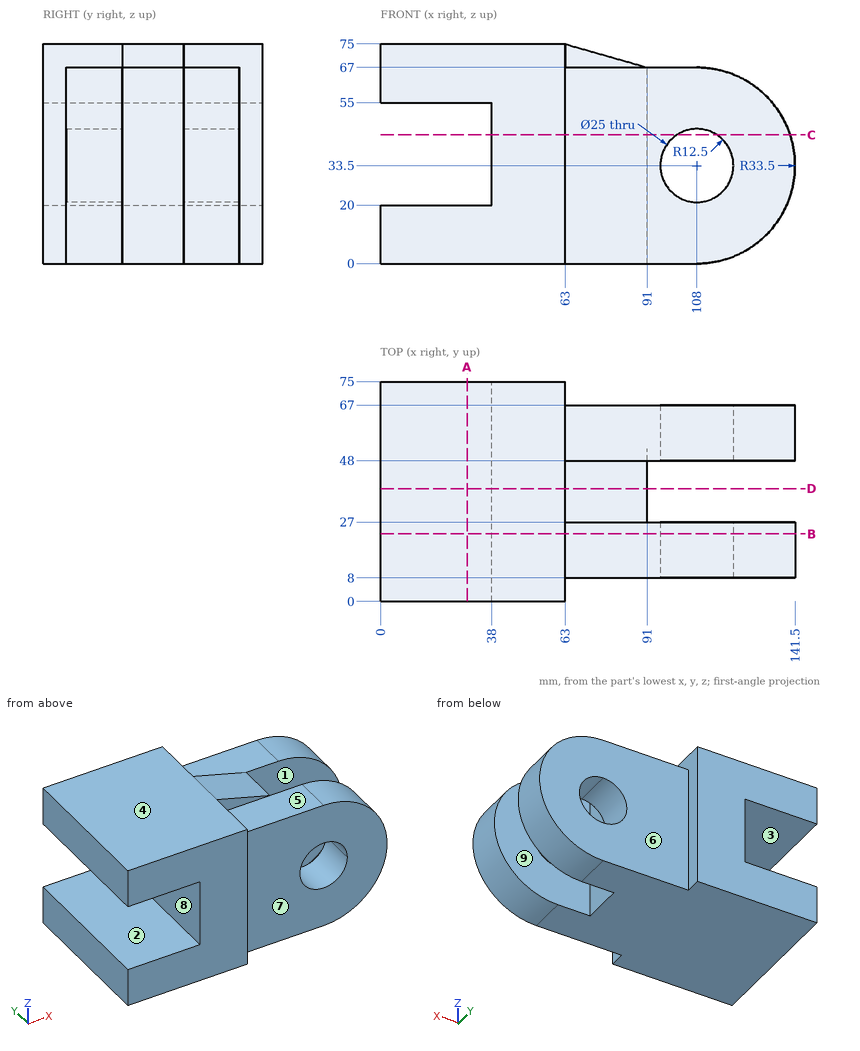
Job drawing, mm, ordinate dimensions from the low corner. One solid piece. A direction names the side the tool comes from. Round coordinates to 2 decimals unless told otherwise and drop trailing zeros. Loops run counter-clockwise (first coordinate to the right, second up) from the corner with the lowest first, then second, coordinate; pieces in that order, holes last.
Item 1: Cut at A-A, the plane x = 29.5. Give the cut face in (y, z), then the cut area to 3 significant figures.
Item 2: Cut at D-D, the plane y = 38.5. Give the cut face in (x, z), then the cut area to 3 significant figures.
Item 3: Mould opens along Z. For the marked faces 1, 2, 3 and 4 say: +Z half, -Z half, draft (parallel to the pull), parting line (faces both ways), or undercut.
Item 4: Drill centre lines: line 1 (Z direction, x = 8, y = 41.5); line 2 (Z direction, x = 108, y = 62); line 3 (Y direction, x = 97, z = 64). Where is each one in solid material? Low to high.
Item 5: Cut at C-C, the plane z = 44. Give the cut face in (x, y), then the cut area to 3 significant figures.
Item 6: Drop flat-ended pins along their axis: P1, Ø6, axis at y = 12, z = 33, coming from the -X side; P2, Ø21.5, axis at y = 65.5, z = 44.5, coming from the +X side; P3, Ø21, axis at x = 88, y = 17, coming from the +Z side; P4, Ø15, axis at x = 108, z = 33.5, coming from the +Y side. Give the stop position or say it passes through.
Item 7: 3-axis set-ups, long thin cutter, end or side, ignore diameter. For the marked faces 5, 6, 7, 8 and 9: which of +Z, -Z, +X, -X, +Y, -Y reach the whole face in a straight line?
Item 8: Cut at B-B, the plane y = 23. Give the cut face in (x, z), then the cut area to 3 significant figures.
A:
1. outline: (0, 0) - (75, 0) - (75, 20) - (0, 20) - close; (0, 55) - (75, 55) - (75, 75) - (0, 75) - close
1. area: 3,000 mm2
2. outline: (0, 0) - (91, 0) - (91, 67) - (63, 75) - (0, 75) - (0, 55) - (38, 55) - (38, 20) - (0, 20) - close
2. area: 5,380 mm2
3. face 1: draft
3. face 2: undercut
3. face 3: undercut
3. face 4: +Z half
4. line 1: z = 0 to 20, 55 to 75
4. line 2: z = 0 to 21, 46 to 67
4. line 3: y = 8 to 27, 48 to 67
5. outline: (38, 0) - (63, 0) - (63, 8) - (101.22, 8) - (101.22, 27) - (91, 27) - (91, 48) - (101.22, 48) - (101.22, 67) - (63, 67) - (63, 75) - (38, 75) - close; (114.78, 8) - (139.81, 8) - (139.81, 27) - (114.78, 27) - close; (114.78, 48) - (139.81, 48) - (139.81, 67) - (114.78, 67) - close
5. area: 4,870 mm2
6. P1: stops at x = 38
6. P2: stops at x = 141.5
6. P3: stops at z = 68.77
6. P4: passes through
7. face 5: +Z, +X, -Y
7. face 6: +Z, -Z, +X, +Y
7. face 7: +Z, -Z, +X, -Y
7. face 8: -X, +Y, -Y
7. face 9: +Z, -Z, +X
8. outline: (0, 0) - (108, 0) arc R33.5 ccw to (108, 67) - (63, 67) - (63, 75) - (0, 75) - (0, 55) - (38, 55) - (38, 20) - (0, 20) - close; hole circle Ø25 at (108, 33.5)
8. area: 7,680 mm2
